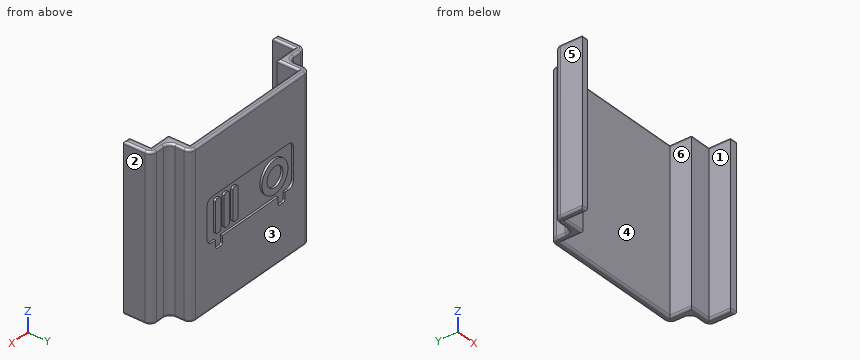
from build123d import *

# Parameters (mm, degrees)
F1_DEPTH = 75
F2_R     = 3
F3_R     = 1
F4_R     = 7.468486
F4_R_2   = 4.590702
F5_DEPTH = 1


with BuildPart() as f1:
    # F0 (on Top) → F1 (new body)
    with BuildSketch(Plane.XY):
        Polygon((-3, 0), (0, 0), (0, 10), (10, 10), (10, 20), (72.5, 20), (72.5, 10), (82.5, 10), (82.5, 0), (86.034332, 0), (86.034332, 13), (76.034332, 13), (76.034332, 23), (7, 23), (7, 13), (-3, 13), align=None)
    extrude(amount=F1_DEPTH)

    # F2
    f2_edges = [f1.edges().sort_by_distance(p)[0] for p in [
        (-3, 13, 37.5),
        (7, 13, 37.5),
        (7, 23, 37.5),
        (76.034332, 23, 37.5),
        (76.034332, 13, 37.5),
        (86.034332, 13, 37.5),
    ]]
    fillet(f2_edges, radius=F2_R)

    # F3
    f3_edges = [f1.edges().sort_by_distance(p)[0] for p in [
        (86.034332, 5, 75),
        (85.155653, 12.12132, 75),
        (84.267166, 0, 75),
        (81.034332, 13, 75),
        (82.5, 5, 75),
        (76.913012, 13.87868, 75),
        (77.5, 10, 75),
        (76.034332, 18, 75),
        (72.5, 15, 75),
        (75.155653, 22.12132, 75),
        (41.25, 20, 75),
        (41.517166, 23, 75),
        (10, 15, 75),
        (7.87868, 22.12132, 75),
        (5, 10, 75),
        (7, 18, 75),
        (0, 5, 75),
        (6.12132, 13.87868, 75),
        (-1.5, 0, 75),
        (2, 13, 75),
        (-3, 5, 75),
        (-2.12132, 12.12132, 75),
        (86.034332, 5, 0),
        (85.155653, 12.12132, 0),
        (84.267166, 0, 0),
        (81.034332, 13, 0),
        (82.5, 5, 0),
        (76.913012, 13.87868, 0),
        (77.5, 10, 0),
        (76.034332, 18, 0),
        (72.5, 15, 0),
        (75.155653, 22.12132, 0),
        (41.25, 20, 0),
        (41.517166, 23, 0),
        (10, 15, 0),
        (7.87868, 22.12132, 0),
        (5, 10, 0),
        (7, 18, 0),
        (0, 5, 0),
        (6.12132, 13.87868, 0),
        (-1.5, 0, 0),
        (2, 13, 0),
        (-3, 5, 0),
        (-2.12132, 12.12132, 0),
    ]]
    fillet(f3_edges, radius=F3_R)

    # F4 (on face) → F5 (cut)
    with BuildSketch(Plane(origin=(0, 23, 0), x_dir=(-1, 0, 0), z_dir=(0, 1, 0))):
        with BuildLine():
            Line((-19.5, 49), (-63.5, 49))
            ThreePointArc((-63.5, 49), (-65.62132, 48.12132), (-66.5, 46))
            Line((-66.5, 46), (-66.5, 32))
            ThreePointArc((-66.5, 32), (-65.62132, 29.87868), (-63.5, 29))
            Line((-63.5, 29), (-61.5, 29))
            Line((-61.5, 29), (-61.5, 26))
            ThreePointArc((-61.5, 26), (-61.207107, 25.292893), (-60.5, 25))
            Line((-60.5, 25), (-58.5, 25))
            ThreePointArc((-58.5, 25), (-57.792893, 25.292893), (-57.5, 26))
            Line((-57.5, 26), (-57.5, 29))
            Line((-57.5, 29), (-25.5, 29))
            Line((-25.5, 29), (-25.5, 26))
            ThreePointArc((-25.5, 26), (-25.207107, 25.292893), (-24.5, 25))
            Line((-24.5, 25), (-22.5, 25))
            ThreePointArc((-22.5, 25), (-21.792893, 25.292893), (-21.5, 26))
            Line((-21.5, 26), (-21.5, 29))
            Line((-21.5, 29), (-19.5, 29))
            ThreePointArc((-19.5, 29), (-17.37868, 29.87868), (-16.5, 32))
            Line((-16.5, 32), (-16.5, 46))
            ThreePointArc((-16.5, 46), (-17.37868, 48.12132), (-19.5, 49))
        make_face()
        with BuildLine():
            ThreePointArc((-61.5, 45.5), (-61.207107, 46.207107), (-60.5, 46.5))
            Line((-60.5, 46.5), (-59.5, 46.5))
            ThreePointArc((-59.5, 46.5), (-58.792893, 46.207107), (-58.5, 45.5))
            Line((-58.5, 45.5), (-58.5, 32.5))
            ThreePointArc((-58.5, 32.5), (-58.792893, 31.792893), (-59.5, 31.5))
            Line((-59.5, 31.5), (-60.5, 31.5))
            ThreePointArc((-60.5, 31.5), (-61.207107, 31.792893), (-61.5, 32.5))
            Line((-61.5, 32.5), (-61.5, 45.5))
        make_face(mode=Mode.SUBTRACT)
        with BuildLine():
            ThreePointArc((-56.5, 45.5), (-56.207107, 46.207107), (-55.5, 46.5))
            Line((-55.5, 46.5), (-54.5, 46.5))
            ThreePointArc((-54.5, 46.5), (-53.792893, 46.207107), (-53.5, 45.5))
            Line((-53.5, 45.5), (-53.5, 32.5))
            ThreePointArc((-53.5, 32.5), (-53.792893, 31.792893), (-54.5, 31.5))
            Line((-54.5, 31.5), (-55.5, 31.5))
            ThreePointArc((-55.5, 31.5), (-56.207107, 31.792893), (-56.5, 32.5))
            Line((-56.5, 32.5), (-56.5, 45.5))
        make_face(mode=Mode.SUBTRACT)
        with BuildLine():
            ThreePointArc((-51.5, 45.5), (-51.207107, 46.207107), (-50.5, 46.5))
            Line((-50.5, 46.5), (-49.5, 46.5))
            ThreePointArc((-49.5, 46.5), (-48.792893, 46.207107), (-48.5, 45.5))
            Line((-48.5, 45.5), (-48.5, 32.5))
            ThreePointArc((-48.5, 32.5), (-48.792893, 31.792893), (-49.5, 31.5))
            Line((-49.5, 31.5), (-50.5, 31.5))
            ThreePointArc((-50.5, 31.5), (-51.207107, 31.792893), (-51.5, 32.5))
            Line((-51.5, 32.5), (-51.5, 45.5))
        make_face(mode=Mode.SUBTRACT)
        with Locations((-27.229397, 38.67811)):
            Circle(F4_R, mode=Mode.SUBTRACT)
        with Locations((-27.229397, 38.67811)):
            Circle(F4_R_2)
    extrude(amount=-F5_DEPTH, mode=Mode.SUBTRACT)


solid = f1.part
Can you work these out from the model? Positions are in its coordinate system, mm. Face numbers are marked on the shaded views. A direction names the side the tool comes from. Coordinates: 2 decimals unless noted, no trailing zeros. Write each loop counter-clockwise with the first axis right and the second up, starting at its lowest first coordinate (ties: lowest second). Pieces come first, ordered by that corner, then holes. Notation, with made-up numbers: (66.5, -27.5) - (102.5, -27.5) arc R13 cw to (102.5, -4.5) - close; hole circle Ø6 at (61.5, 52). An arc over 180 degrees is marked (long way). Return JSON: item names as keys, results as strings. Group by question number.
Item 1: If we section it at B-B (x = 13): Write out the boundary of the cut face in (y, z), then the cut area to 3 significant figures.
Item 2: If we section it at A-A (y = 17.75): Write out the boundary of the cut face in (x, z).
Item 3: We'd pull the mould along X, two halves only. Please class the marked faces 3, 4, 5 and 6: pulls with the +X half, pulls with the -X half, needs draft (parallel to the pull), parting line crosses it, or undercut.
Item 4: Please list where these lines run through material, in increasing order: probe 1 along X at (y, z) = (6.25, 52); probe 2 along X at (y, z) = (17.75, 12.5); probe 3 along Y at (x, z) = (64, 11).
Item 5: If we section it at D-D (x = 38.5): Write out the boundary of the cut face in (y, z), then the cut area to 3 significant figures.
Item 6: I'm going to push flat-ended pins straight in: pin 1 Ø1.5 at (x, z) = (20.5, 32) entering from -Y; pin 2 Ø3 at (y, z) = (13.5, 24) entering from -X; pin 3 Ø4.5 at (y, z) = (17, 24.5) entering from +X. Where does each tip first touch, or does it pass through?
Item 7: Which directions (+Z, -Z, +X, -X, +Y, -Y) give clear straight access to the entire face, cutting with the end or side of a thin tool? Please do the marked faces 1 and 2.
Item 8: If we section it at C-C (z = 59): Write out the boundary of the cut face in (x, y).
Return value:
{
 "1": {"outline": "(20, 1) arc R1 ccw to (21, 0) - (22, 0) arc R1 ccw to (23, 1) - (23, 74) arc R1 ccw to (22, 75) - (21, 75) arc R1 ccw to (20, 74) - close", "area": "224 mm^2"},
 "2": {"outline": "(7, 1) arc R1 ccw to (8, 0) - (9, 0) arc R1 ccw to (10, 1) - (10, 74) arc R1 ccw to (9, 75) - (8, 75) arc R1 ccw to (7, 74) - close; (72.5, 1) arc R1 ccw to (73.5, 0) - (75.03, 0) arc R1 ccw to (76.03, 1) - (76.03, 74) arc R1 ccw to (75.03, 75) - (73.5, 75) arc R1 ccw to (72.5, 74) - close"},
 "3": {"face 3": "needs draft", "face 4": "undercut", "face 5": "pulls with the -X half", "face 6": "undercut"},
 "4": {"probe 1": "x = -3 to 0, 82.5 to 86.03", "probe 2": "x = 7 to 10, 72.5 to 76.03", "probe 3": "y = 20 to 23"},
 "5": {"outline": "(20, 1) arc R1 ccw to (21, 0) - (22, 0) arc R1 ccw to (23, 1) - (23, 29) - (22, 29) - (22, 49) - (23, 49) - (23, 74) arc R1 ccw to (22, 75) - (21, 75) arc R1 ccw to (20, 74) - close", "area": "204 mm^2"},
 "6": {"pin 1": "stops at y = 20", "pin 2": "stops at x = -2.24", "pin 3": "stops at x = 76.31"},
 "7": {"face 1": "+Z, -Z, -Y", "face 2": "+Z, -Z, +X, +Y, -Y"},
 "8": {"outline": "(-3, 0) - (0, 0) - (0, 10) - (10, 10) - (10, 20) - (72.5, 20) - (72.5, 10) - (82.5, 10) - (82.5, 0) - (86.03, 0) - (86.03, 10) arc R3 ccw to (83.03, 13) - (79.03, 13) arc R3 cw to (76.03, 16) - (76.03, 20) arc R3 ccw to (73.03, 23) - (10, 23) arc R3 ccw to (7, 20) - (7, 16) arc R3 cw to (4, 13) - (0, 13) arc R3 ccw to (-3, 10) - close"}
}
